Design review of the part built by this model. Coordinates are the model's own, in mm. Face numbers are marked on the shaded views. A direction names the side the tool comes from. Round coordinates to 2 decimals unless told otherwise and drop trailing zeros. Order: outer loops, then holes, each group sorted by start corner. A loop starts at its lowest first (then second) coordinate and runs counter-clockwise, first axis right, second up. Notation, with made-up numbers: M 30,87.5 L 41,87.5 A22 ccw 41,116.5 Z; hole C -39,-20.5 d7. An arc over 180 degrees is marked long. Use a Markdown table: item, result. Add a question column.
(1) For pin 1 (10 mm diameter, centred on x = 55, z = 84, fed in from -Y); pin 2 (10 mm diameter, centred on x = 57, z = 75.5, fed in from +Y); pin 3 (1 mm diameter, centred on x = 43.5, y = 29, fed in from +Z), all flat-tipped, find the tip position at first contact; note any pin that passes through.
(2) Machinability: for the marked faces 1, 2, 3 and 4, which of the approach directions +Z, -Z, +X, -X, +Y, -Y give a long, thin tool a straight path to every point of the face, cutting with its end or side? Answer none if there is none.
(3) Take a section at A-A (z = 77.5). Write out the cut boundary in (x, y), then the cut area to 3 significant figures.
(4) The part is to be moulded in two halves that separate along X. For the marked faces 5, 6 and 7, say which applies: released by +X, released by -X, zero draft, split by the parting line, or undercut.
(5) Take a section at D-D (z = 56.5). Write out the cut boundary in (x, y).
(6) Take a section at B-B (y = 57). Write out the cut boundary in (x, z).
(7) To check wall thickness, follow probe 1 along X at (y, z) = (67, 30.5); probe 2 along Y at (x, z) = (104.5, 73.5). State the ranges of each line that lie inside material, in increasing order. Write a range as from..to.
```python
from build123d import *

# Parameters (mm, degrees)
ESQUISSE1_W             = 120
ESQUISSE1_H             = 120
BOSS_EXTRU_1_DEPTH      = 90
CONG_1_R                = 5
COQUE1_T                = -2
ENL_V_MAT_EXTRU_2_DEPTH = 20


with BuildPart() as part:
    # Esquisse1 → Boss.-Extru.1 (new body)
    with BuildSketch(Plane.XY):
        with Locations((60, 60)):
            Rectangle(ESQUISSE1_W, ESQUISSE1_H)
    extrude(amount=BOSS_EXTRU_1_DEPTH)

    # Congé1
    cong_1_edges = [part.edges().sort_by_distance(p)[0] for p in [
        (0, 120, 45),
        (120, 120, 45),
        (120, 0, 45),
        (0, 0, 45),
    ]]
    fillet(cong_1_edges, radius=CONG_1_R)

    # Coque1
    coque1_openings = [part.faces().sort_by_distance(p)[0] for p in [
        (60, 60, 90),
    ]]
    offset(amount=COQUE1_T, openings=coque1_openings, kind=Kind.INTERSECTION)

    # Esquisse4 → Enlèv. mat.-Extru.2 (cut)
    with BuildSketch(Plane.XY.offset(90)):
        with BuildLine():
            Line((0, 115), (0, 5))
            ThreePointArc((0, 5), (1.464466094, 1.464466094), (5, 0))
            Line((5, 0), (115, 0))
            ThreePointArc((115, 0), (118.535533906, 1.464466094), (120, 5))
            Line((120, 5), (120, 115))
            ThreePointArc((120, 115), (118.535533906, 118.535533906), (115, 120))
            Line((115, 120), (5, 120))
            ThreePointArc((5, 120), (1.464466094, 118.535533906), (0, 115))
        make_face()
        with BuildLine():
            Line((1, 115), (1, 5))
            ThreePointArc((1, 5), (2.171572875, 2.171572875), (5, 1))
            Line((5, 1), (115, 1))
            ThreePointArc((115, 1), (117.828427125, 2.171572875), (119, 5))
            Line((119, 5), (119, 115))
            ThreePointArc((119, 115), (117.828427125, 117.828427125), (115, 119))
            Line((115, 119), (5, 119))
            ThreePointArc((5, 119), (2.171572875, 117.828427125), (1, 115))
        make_face(mode=Mode.SUBTRACT)
    extrude(amount=-ENL_V_MAT_EXTRU_2_DEPTH, mode=Mode.SUBTRACT)


solid = part.part
```
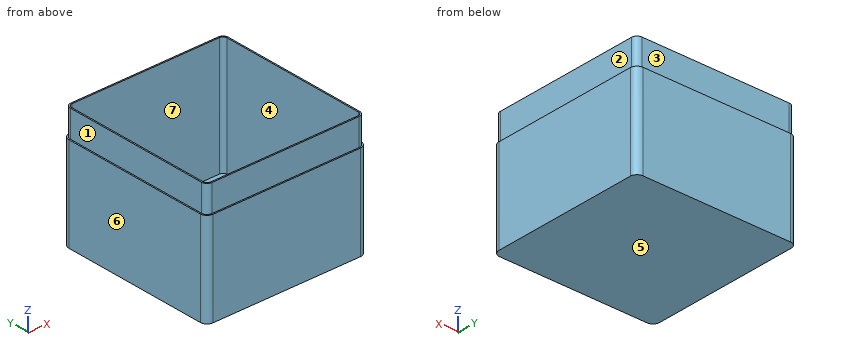
Verdict:
| question | item | result |
|---|---|---|
| 1 | pin 1 | stops at y = 1 |
| 1 | pin 2 | stops at y = 119 |
| 1 | pin 3 | stops at z = 2 |
| 2 | face 1 | +Z, -X, +Y, -Y |
| 2 | face 2 | +Z, +X, +Y, -Y |
| 2 | face 3 | +Z, +X, -X, +Y |
| 2 | face 4 | +Z |
| 3 | outline | M 1,5 A4 ccw 5,1 L 115,1 A4 ccw 119,5 L 119,115 A4 ccw 115,119 L 5,119 A4 ccw 1,115 Z; hole M 2,5 A3 ccw 5,2 L 115,2 A3 ccw 118,5 L 118,115 A3 ccw 115,118 L 5,118 A3 ccw 2,115 Z |
| 3 | area | 462 mm^2 |
| 4 | face 5 | zero draft |
| 4 | face 6 | released by -X |
| 4 | face 7 | undercut |
| 5 | outline | M 0,5 A5 ccw 5,0 L 115,0 A5 ccw 120,5 L 120,115 A5 ccw 115,120 L 5,120 A5 ccw 0,115 Z; hole M 2,5 A3 ccw 5,2 L 115,2 A3 ccw 118,5 L 118,115 A3 ccw 115,118 L 5,118 A3 ccw 2,115 Z |
| 6 | outline | M 0,0 L 120,0 L 120,70 L 119,70 L 119,90 L 118,90 L 118,2 L 2,2 L 2,90 L 1,90 L 1,70 L 0,70 Z |
| 7 | probe 1 | x = 0..2, 118..120 |
| 7 | probe 2 | y = 1..2, 118..119 |
